Input: part model. Units: mm. Frame: model coordinates. A direction names the side the tool comes from. Give positions to 0.01 mm unless a question says otherwise; leave off trailing zeros. Write each loop counter-clockwise with the first axis right and the second up, starting at its lowest first coordinate (ties: lowest second). Pieces come first, ordered by that corner, then holes. Notation, with made-up numbers: (76.5, 24) -> (80.5, 24) arc R31 ccw to (80.5, 52) -> close; hole circle Ø10 at (43, -10.75). An arc over 180 degrees is marked (long way). Return JSON: item names as keys, results as strings. Group by question number.
Item 1: Pin query (flat end, axial travel): P1, Ø5, axis at x = 4.5, z = 10.5, coming from the -Y side; P2, Ø1.5, axis at y = 3.5, z = 10.5, coming from the -X side; P3, Ø1.7, axis at x = 2.5, y = -1, coming from the -Z side; P4, Ø4.5, axis at y = 1, z = 6, coming from the +X side. Return the tip coordinate at first contact, or that it passes through.
Item 2: Section C-C, the plane x = 0. Return loops of the section in (y, z).
Item 3: Line query: line 1 (Y direction, x = 0, z = 1.75); line 2 (Y direction, x = 0, z = 3.3); line 3 (Z direction, x = -5, y = 0). Output: solid intervals per line, ascending. Write a range as [from, to].
Item 4: Mould query, pull axis Y, two halves, no side actions, for faces 1 (the face through (3.15, 0.04, 7.06)), 2 (the face through (-6.24, 3.17, 5.05)), 3 (the face through (1.102, -6.913, 5.053)), 4 (the face through (0, 0, 12)). Classes: released by +Y, released by -Y, zero draft, split by the parting line, or undercut.
Item 5: Section A-A, the plane z = 6. Return loops of the section in (x, y).
Item 6: Section B-B, the plane y = 0. Return loops of the section in (x, z), then the cut area to 3 significant figures.
Item 7: Set-up query: faces 5 (the face through (-6.915, 1.088, 5.053)), 6 (the face through (3, -3, 2.4)). Return all of +Z, -Z, +X, -X, +Y, -Y with unobstructed straight access to the full face (end or side cutting, diameter ignored); none if empty.
Autodesk Fusion 360 part; units mm, degrees
sketch "Sketch1" plane through (0, 0, 0) normal (0, 0, 1) x (1, 0, 0)
  circle A0 centre (0, 0) radius 7
  dimension "d1" = 14
extrude "Extrude1" add sketch "Sketch1" along normal blind 12
fillet "Fillet1" radius 1.75 1 edges at (-6.5263, -2.5313, 12)
sketch "Sketch2" plane through (0, 0, 0) normal (0, 0, -1) x (1, 0, 0)
  circle A0 centre (0, 0) radius 7
  circle A1 centre (0, 0) radius 7
  circle A2 centre (0, 0) radius 6
  circle A3 centre (0, 0) radius 7
  line L0 (0, 0) -> (0, 0.2) construction
  line L1 (0, 0.2) -> (0, 7) construction
  line L2 (0, 6) -> (0.65, 6) construction
  line L3 (0, 7) -> (0.6591, 6.9689) construction
  line L4 (0.65, 6) -> (0.65, 6.9845) construction
  line L5 (0.65, 6.4922) -> (0, 6.4922) construction
  circle A4 centre (0, 7) radius 0.5657
  circle A5 centre (-2.1631, 6.6574) radius 0.5657
  circle A6 centre (-4.1145, 5.6631) radius 0.5657
  circle A7 centre (-5.6631, 4.1145) radius 0.5657
  circle A8 centre (-6.6574, 2.1631) radius 0.5657
  circle A9 centre (-7, 0) radius 0.5657
  circle A10 centre (-6.6574, -2.1631) radius 0.5657
  circle A11 centre (-5.6631, -4.1145) radius 0.5657
  circle A12 centre (-4.1145, -5.6631) radius 0.5657
  circle A13 centre (-2.1631, -6.6574) radius 0.5657
  circle A14 centre (0, -7) radius 0.5657
  circle A15 centre (2.1631, -6.6574) radius 0.5657
  circle A16 centre (4.1145, -5.6631) radius 0.5657
  circle A17 centre (5.6631, -4.1145) radius 0.5657
  circle A18 centre (6.6574, -2.1631) radius 0.5657
  circle A19 centre (7, 0) radius 0.5657
  circle A20 centre (6.6574, 2.1631) radius 0.5657
  circle A21 centre (5.6631, 4.1145) radius 0.5657
  circle A22 centre (4.1145, 5.6631) radius 0.5657
  circle A23 centre (2.1631, 6.6574) radius 0.5657
  dimension "d6" = 1
  dimension "d8" = 360
extrude "Extrude2" cut sketch "Sketch2" against normal up to surface (12 mm away) contours A0 A1 A3 A19 | A0 A1 A3 A20 | A0 A1 A3 A18 | A0 A1 A3 A21 | A0 A1 A3 A17 | A0 A1 A3 A22 | A0 A1 A3 A16 | A0 A1 A3 A23 | A0 A1 A3 A15 | A0 A1 A3 A4 | A0 A1 A3 A14 | A0 A1 A3 A5 | A0 A1 A3 A13 | A0 A1 A3 A6 | A0 A1 A3 A12 | A0 A1 A3 A7 | A0 A1 A3 A11 | A0 A1 A3 A8 | A0 A1 A3 A10 | A0 A1 A3 A9 picked at (7.1797, -0.1173) picked at (6.8361, 2.2176) picked at (6.8361, -2.2176) picked at (5.5015, 4.0141) picked at (5.8177, -4.2195) picked at (4.0141, 5.5015) picked at (4.2165, -5.8197) picked at (2.0914, 6.4812) picked at (2.2148, -6.837) picked at (-0.0137, 6.8102) picked at (-0.0038, -7.1868) picked at (-2.2209, 6.8351) picked at (-2.1158, -6.4731) picked at (-4.2243, 5.8143) picked at (-3.9923, -5.5173) picked at (-5.8143, 4.2243) picked at (-5.5036, -4.0109) picked at (-6.4748, 2.1098) picked at (-6.4748, -2.1098) picked at (-6.8097, 0)
sketch "Sketch3" plane through (0, 0, 0) normal (0, 0, 1) x (1, 0, 0)
  circle A0 centre (0, 0) radius 6
  dimension "d11" = 12
extrude "Extrude3" cut sketch "Sketch3" along normal blind 2.4
sketch "Sketch4" plane through (0, 0, 2.4) normal (0, 0, -1) x (1, 0, 0)
  circle A0 centre (0, 0) radius 6
  circle A1 centre (0, 0) radius 3.5
  dimension "d14" = 7
extrude "Extrude4" cut sketch "Sketch4" against normal blind 1.8 contours A1
sketch "Sketch5" plane through (0, 0, 4.2) normal (0, 0, -1) x (1, 0, 0)
  circle A0 centre (0, 0) radius 3.5
  circle A1 centre (0, 0) radius 3.5
  circle A2 centre (0, 0) radius 3.15
  line L0 (1.65, 4.5) -> (1.65, -4.3)
  line L1 (3.15, 4.1) -> (3.15, -3.8) construction
  dimension "d17" = 6.3
  dimension "d18" = 1.5
extrude "Extrude5" cut sketch "Sketch5" against normal up to surface (5.8 mm away) contours A2 L0 picked at (1.774, -0.8051)
Answer below:
{
 "1": {"P1": "stops at y = -6.46", "P2": "stops at x = -6.43", "P3": "stops at z = 2.4", "P4": "stops at x = 7"},
 "2": {"outline": "(-6.43, 0) -> (-6, 0) -> (-6, 2.4) -> (-3.5, 2.4) -> (-3.5, 4.2) -> (3.5, 4.2) -> (3.5, 2.4) -> (6, 2.4) -> (6, 0) -> (7, 0) -> (7, 10.25) arc R1.75 ccw to (5.25, 12) -> (-5.25, 12) arc R1.75 ccw to (-6.43, 11.54) -> close"},
 "3": {"line 1": "y = [-6.43, -6], [6, 7]", "line 2": "y = [-6.43, -3.5], [3.5, 7]", "line 3": "z = [2.4, 12]"},
 "4": {"face 1": "undercut", "face 2": "released by +Y", "face 3": "released by -Y", "face 4": "zero draft"},
 "5": {"outline": "(-6.98, -0.57) arc R7 ccw to (-6.81, -1.62) arc R0.57 cw to (-6.46, -2.69) arc R7 ccw to (-0.57, -6.98) arc R0.57 cw to (0.57, -6.98) arc R7 ccw to (1.62, -6.81) arc R0.57 cw to (2.69, -6.46) arc R7 ccw to (3.64, -5.98) arc R0.57 cw to (4.56, -5.31) arc R7 ccw to (5.31, -4.56) arc R0.57 cw to (5.98, -3.64) arc R7 ccw to (-1.62, 6.81) arc R0.57 cw to (-2.69, 6.46) arc R7 ccw to (-3.64, 5.98) arc R0.57 cw to (-4.56, 5.31) arc R7 ccw to (-5.31, 4.56) arc R0.57 cw to (-5.98, 3.64) arc R7 ccw to (-6.46, 2.69) arc R0.57 cw to (-6.81, 1.62) arc R7 ccw to (-6.98, 0.57) arc R0.57 cw to start; hole (1.65, -2.68) arc R3.15 ccw to (1.65, 2.68) -> close"},
 "6": {"outline": "(-6.43, 0) -> (-6, 0) -> (-6, 2.4) -> (-3.5, 2.4) -> (-3.5, 4.2) -> (1.65, 4.2) -> (1.65, 10) -> (3.15, 10) -> (3.15, 4.2) -> (3.5, 4.2) -> (3.5, 2.4) -> (6, 2.4) -> (6, 0) -> (7, 0) -> (7, 10.25) arc R1.75 ccw to (5.25, 12) -> (-5.25, 12) arc R1.75 ccw to (-6.43, 11.54) -> close", "area": "110 mm2"},
 "7": {"face 5": "+Z, -Z, -X, +Y", "face 6": "-Z"}
}
